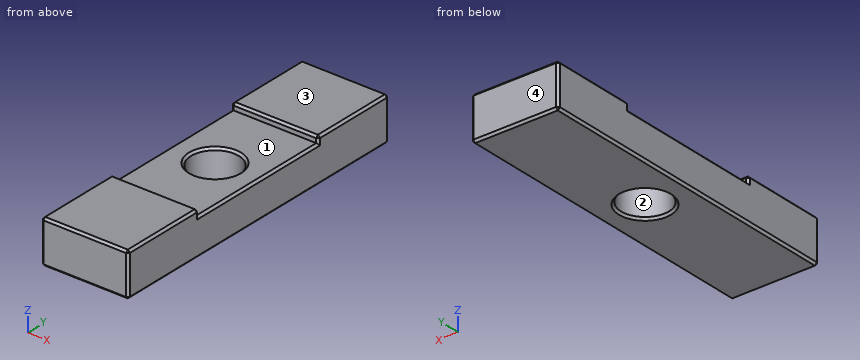
```python
from build123d import *

# Parameters (mm, degrees)
F0_W     = 20
F0_H     = 74
F1_DEPTH = 10
F2_W     = 20
F2_H     = 34
F3_DEPTH = 1.5
F4_R     = 5.5
F5_DEPTH = 8.501
F6_SIZE  = 0.5


with BuildPart() as f1:
    # F0 (on Top) → F1 (new body)
    with BuildSketch(Plane.XY):
        Rectangle(F0_W, F0_H)
    extrude(amount=F1_DEPTH)

    # F2 (on face) → F3 (cut)
    with BuildSketch(Plane.XY.offset(10)):
        Rectangle(F2_W, F2_H)
    extrude(amount=-F3_DEPTH, mode=Mode.SUBTRACT)

    # F4 (on face) → F5 (cut, through all)
    with BuildSketch(Plane.XY.offset(8.5)):
        Circle(F4_R)
    extrude(amount=-F5_DEPTH, mode=Mode.SUBTRACT)

    # F6
    f6_edges = [f1.edges().sort_by_distance(p)[0] for p in [
        (-5.5, 0, 8.5),
        (10, -37, 5),
        (-10, -37, 5),
        (10, 37, 5),
        (-10, 37, 5),
        (-10, 0, 0),
        (0, -37, 0),
        (10, 0, 0),
        (0, 37, 0),
        (10, 27, 10),
        (-10, 27, 10),
        (-10, -27, 10),
        (10, -27, 10),
        (10, 0, 8.5),
        (-10, 0, 8.5),
        (0, 37, 10),
        (0, -37, 10),
        (-5.5, 0, 0),
        (0, 17, 10),
        (0, -17, 10),
        (-10, -17, 9.25),
        (-10, 17, 9.25),
        (10, 17, 9.25),
        (10, -17, 9.25),
    ]]
    chamfer(f6_edges, length=F6_SIZE)


solid = f1.part
```
The listing builds one solid part. Answer for the finished solid, in the listing's coordinates (mm). Face numbers are marked on the shaded views. Give positions to 0.01 mm unless a question says otherwise; leave off trailing zeros. Loops run counter-clockwise (first coordinate to the right, second up) from the corner with the lowest first, then second, coordinate; pieces in that order, holes last. Notation, with made-up numbers: M -2,5 L 44,5 A20 cw 44,30 Z; hole C 15,-19 d7. An arc over 180 degrees is marked long. One line per item, written item: value.
Q1. Determine the mould class of the marked faces 1, 2, 3 and 4 for opening direction Y: +Y half, -Y half, draft (parallel to the pull), parting line (faces both ways), or undercut.
Working result:
face 1: undercut
face 2: undercut
face 3: draft
face 4: +Y half
Q2. A cutting plane is placed at D-D on y = 9. Determine the outline of the cut face in (x, z), then the cut area to 4 significant figures.
Working result:
outline: M -10,0.5 L -9.5,0 L 9.5,0 L 10,0.5 L 10,8 L 9.5,8.5 L -9.5,8.5 L -10,8 Z
area: 169.5 mm^2
Q3. A cutting plane is placed at A-A on y = 0. Determine the outline of the cut face in (x, z).
Working result:
outline: M -10,0.5 L -9.5,0 L -6,0 L -5.5,0.5 L -5.5,8 L -6,8.5 L -9.5,8.5 L -10,8 Z; M 5.5,0.5 L 6,0 L 9.5,0 L 10,0.5 L 10,8 L 9.5,8.5 L 6,8.5 L 5.5,8 Z
Q4. A flat-ended cylindrical pin translates along its axis: P1, Ø9.5, axis at x = 3, y = 5.5, coming from the +Z side. Find the tip coordinate at first contact, or state that the pin passes through.
Working result:
P1: stops at z = 8.5
Q5. Find the intervals of material crossed by line 1 (Y direction, x = 0, z = 6); line 2 (Z direction, x = 6.5, y = -4.5); line 3 (Y direction, x = -4.25, z = 4.75), in increasing order. Write a range as from..to.
Working result:
line 1: y = -37..-5.5, 5.5..37
line 2: z = 0..8.5
line 3: y = -37..-3.49, 3.49..37
Q6. A cutting plane is placed at C-C on x = 0. Determine the outline of the cut face in (y, z), then the cut area to 3 significant figures.
Working result:
outline: M -37,0.5 L -36.5,0 L -6,0 L -5.5,0.5 L -5.5,8 L -6,8.5 L -17,8.5 L -17,9.5 L -17.5,10 L -36.5,10 L -37,9.5 Z; M 5.5,0.5 L 6,0 L 36.5,0 L 37,0.5 L 37,9.5 L 36.5,10 L 17.5,10 L 17,9.5 L 17,8.5 L 6,8.5 L 5.5,8 Z
area: 594 mm^2
Q7. A cutting plane is placed at B-B on z = 4.25. Determine the outline of the cut face in (x, y).
Working result:
outline: M -10,-36.5 L -9.5,-37 L 9.5,-37 L 10,-36.5 L 10,36.5 L 9.5,37 L -9.5,37 L -10,36.5 Z; hole C 0,0 d11
